Model file for the job. Use its own axes, mm. A direction names the side the tool comes from. Round coordinates to 2 decimals unless told otherwise and drop trailing zeros. Loops run counter-clockwise (first coordinate to the right, second up) from the corner with the lowest first, then second, coordinate; pieces in that order, holes last. Notation, with made-up numbers: M 36.5,77.25 L 74.5,77.25 A32 cw 74.5,114.25 Z; hole C 62,69 d9. An arc over 180 degrees is marked long. Use a Markdown table: item, result. Add a question column.
Q1. Cut at D-D (z = 0). Give the cut face in (x, y).
Q2. Cut at A-A (z = 89). Give the cut face in (x, y).
Q3. Cut at C-C (x = 0). Give the cut face in (y, z).
Q4. Mould opens along Y. For faces 1 (the face through (2, 254, 2)), 2 (the face through (32, 247.65, 32)), 3 (the face through (-127.192, 250.781, 40.055)), 4 (the face through (-2, 0, 2)) say: +Y half, -Y half, draft (parallel to the pull), parting line (faces both ways), or undercut.
Q5. Tool access for faces 5 (the face through (-42.397, 125.311, 13.352)), 6 (the face through (127.192, 3.131, 40.055)): list every direction of +Z, -Z, +X, -X, +Y, -Y with a clear straight run to the whole face (end or side of a thin tool).
Q6. Cut at B-B (x = 91.5). Give the cut face in (y, z), plus the area to 3 significant figures.
Q7. Pin check, flat tips, straight feed: pin 1 (12 mm diameter, centred on y = 214, z = 24.5, fed in from -X); pin 2 (6 mm diameter, centred on x = 18, y = 183, fed in from +Z); pin 3 (10 mm diameter, centred on x = -26, y = 122, fed in from +Z). Stop position of each tip, or through.
Q8. Probe line 1 (Y direction, x = 64, z = -73.5); line 2 (X direction, y = 97, z = -4.5); line 3 (X direction, y = 105, z = -33). List the from-to ranges inside material, lowest first. Write a range as from..to.
from build123d import *

# Parameters (mm, degrees)
F0_R     = 133.35
F1_DEPTH = 6.35
F2_R     = 44.45
F3_DEPTH = 241.3
F4_R     = 133.35
F4_R_2   = 44.45
F5_DEPTH = 6.35


with BuildPart() as f1:
    # F0 (on Front) → F1 (new body)
    with BuildSketch(Plane.XZ):
        Circle(F0_R)
    extrude(amount=-F1_DEPTH)

    # F2 (on face) → F3 (join)
    with BuildSketch(Plane(origin=(0, 6.35, 0), x_dir=(-1, 0, 0), z_dir=(0, 1, 0))):
        Circle(F2_R)
    extrude(amount=F3_DEPTH)

    # F4 (on face) → F5 (join)
    with BuildSketch(Plane(origin=(0, 247.65, 0), x_dir=(-1, 0, 0), z_dir=(0, 1, 0))):
        Circle(F4_R)
        Circle(F4_R_2, mode=Mode.SUBTRACT)
        Circle(F4_R_2)
    extrude(amount=F5_DEPTH)


solid = f1.part
Checked values:
| question | item | result |
|---|---|---|
| 1 | outline | M -133.35,0 L 133.35,0 L 133.35,6.35 L 44.45,6.35 L 44.45,247.65 L 133.35,247.65 L 133.35,254 L -133.35,254 L -133.35,247.65 L -44.45,247.65 L -44.45,6.35 L -133.35,6.35 Z |
| 2 | outline | M -99.3,0 L 99.3,0 L 99.3,6.35 L -99.3,6.35 Z; M -99.3,247.65 L 99.3,247.65 L 99.3,254 L -99.3,254 Z |
| 3 | outline | M 0,-133.35 L 6.35,-133.35 L 6.35,-44.45 L 247.65,-44.45 L 247.65,-133.35 L 254,-133.35 L 254,133.35 L 247.65,133.35 L 247.65,44.45 L 6.35,44.45 L 6.35,133.35 L 0,133.35 Z |
| 4 | face 1 | +Y half |
| 4 | face 2 | undercut |
| 4 | face 3 | draft |
| 4 | face 4 | -Y half |
| 5 | face 5 | none |
| 5 | face 6 | +Y, -Y |
| 6 | outline | M 0,-97.01 L 6.35,-97.01 L 6.35,97.01 L 0,97.01 Z; M 247.65,-97.01 L 254,-97.01 L 254,97.01 L 247.65,97.01 Z |
| 6 | area | 2,460 mm^2 |
| 7 | pin 1 | stops at x = -40.42 |
| 7 | pin 2 | stops at z = 41.84 |
| 7 | pin 3 | stops at z = 39.18 |
| 8 | line 1 | y = 0..6.35, 247.65..254 |
| 8 | line 2 | x = -44.22..44.22 |
| 8 | line 3 | x = -29.78..29.78 |
